from build123d import *

# Parameters (mm, degrees)
F0_R     = 4.1529
F1_DEPTH = 6.35
F2_R     = 5.08
F3_R     = 0.79375
F4_DEPTH = 6.604


with BuildPart() as f1:
    # F0 (on Top) → F1 (new body)
    with BuildSketch(Plane.XY):
        with BuildLine():
            Line((-39.5852921817, 35.7330972108), (-43.6584469102, 37.7552635994))
            ThreePointArc((-43.6584469102, 37.7552635994), (-77.757072432, 20.950769545), (-57.9630675112, -11.5038857774))
            Line((-57.9630675112, -11.5038857774), (-52.1653779445, -11.9667752425))
            ThreePointArc((-52.1653779445, -11.9667752425), (-34.5169287333, -4.1314539733), (-27.2771428081, 13.7695381418))
            ThreePointArc((-27.2771428081, 13.7695381418), (-30.5639418609, 26.3581090295), (-39.5852921817, 35.7330972108))
        make_face()
        with BuildLine():
            ThreePointArc((-39.5852921817, 35.7330972108), (-41.5771437171, 36.8342695403), (-43.6584469102, 37.7552635994))
            Line((-43.6584469102, 37.7552635994), (-39.5852921817, 35.7330972108))
        make_face()
        with BuildLine():
            Line((-52.1653779445, -11.9667752425), (-57.9630675112, -11.5038857774))
            ThreePointArc((-57.9630675112, -11.5038857774), (-55.0773333512, -11.8995410396), (-52.1653779445, -11.9667752425))
        make_face()
        with BuildLine():
            Line((0, 16.0805053817), (-39.5852921817, 35.7330972108))
            ThreePointArc((-39.5852921817, 35.7330972108), (-30.5639418609, 26.3581090295), (-27.2771428081, 13.7695381418))
            ThreePointArc((-27.2771428081, 13.7695381418), (-34.5169287333, -4.1314539733), (-52.1653779445, -11.9667752425))
            Line((-52.1653779445, -11.9667752425), (-1.2798007555, -16.0294966658))
            ThreePointArc((-1.2798007555, -16.0294966658), (-16.0677481424, 0.6404084366), (0, 16.0805053817))
        make_face()
        with BuildLine():
            ThreePointArc((12.550681619, 10.0530116996), (6.9615064675, 14.4955193434), (0, 16.0805053817))
            ThreePointArc((0, 16.0805053817), (-16.0677481424, 0.6404084366), (-1.2798007555, -16.0294966658))
            ThreePointArc((-1.2798007555, -16.0294966658), (10.9087765216, -11.8144508181), (16.0805053817, 0))
            ThreePointArc((16.0805053817, 0), (15.91872127, 2.2752948071), (15.4366243175, 4.5048066565))
            ThreePointArc((15.4366243175, 4.5048066565), (12.8528968999, 6.6855358941), (12.550681619, 10.0530116996))
        make_face()
        Circle(F0_R, mode=Mode.SUBTRACT)
        with BuildLine():
            ThreePointArc((21.2413206768, 8.7367389351), (17.4619629936, 13.1316161013), (12.550681619, 10.0530116996))
            ThreePointArc((12.550681619, 10.0530116996), (14.2659723887, 7.4205582766), (15.4366243175, 4.5048066565))
            ThreePointArc((15.4366243175, 4.5048066565), (19.4149247594, 5.1449514054), (21.2413206768, 8.7367389351))
        make_face()
        with BuildLine():
            ThreePointArc((15.4366243175, 4.5048066565), (14.2659723887, 7.4205582766), (12.550681619, 10.0530116996))
            ThreePointArc((12.550681619, 10.0530116996), (12.8528968999, 6.6855358941), (15.4366243175, 4.5048066565))
        make_face()
    extrude(amount=F1_DEPTH)

    # F2
    f2_edges = [f1.edges().sort_by_distance(p)[0] for p in [
        (12.550682, 10.053012, 3.175),
        (15.436624, 4.504807, 3.175),
        (0, 16.080505, 3.175),
    ]]
    fillet(f2_edges, radius=F2_R)

    # F3 (on face) → F4 (cut)
    with BuildSketch(Plane.XY.offset(6.35)):
        with Locations((16.7963206768, 8.7367389351)):
            Circle(F3_R)
    extrude(amount=-F4_DEPTH, mode=Mode.SUBTRACT)


solid = f1.part
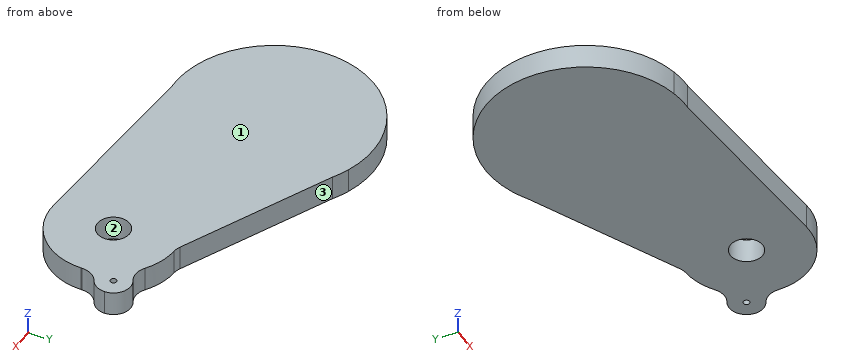
For this review, take the finished solid that the model builds, in its own axes (mm). Face numbers are marked on the shaded views. Give positions to 0.01 mm unless a question says otherwise; leave off trailing zeros. Order: outer loops, then holes, each group sorted by start corner. A loop starts at its lowest first (then second) coordinate and runs counter-clockwise, first axis right, second up. Notation, with made-up numbers: M 26.25,52.25 L 64.25,52.25 A25 ccw 64.25,86.25 Z; hole C 3,31.25 d9. An arc over 180 degrees is marked long. Answer in a Markdown table with one row per item. Add a question column.
(1) Consider section C-C on y = 28. State the section outline as (x, z) points.
(2) Consider section D-D on x = -50.5. State the section outline as (y, z) points.
(3) Wall thickness on probe 1 along X at (y, z) = (-3.5, 2.75); probe 2 along X at (y, z) = (12.5, 1.5); probe 3 along Y at (x, z) = (0, 1.5): over which ranges is each line inside the solid? List them lowest first. Write a range as [from, to].
(4) Mouldability with a two-part tool opening along X and no side actions: class the marked faces 1, 2 and 3 as +X half, -X half, draft (parallel to the pull), parting line (faces both ways), or undercut.
(5) Consider section A-A on x = 0. State the section outline as (y, z) points, and give its area (3 significant figures).
(6) For pin 1 (1.4 mm diameter, centred on x = 16.8, y = 8.74, fed in from +Z); pin 2 (3 mm diameter, centred on x = -15.5, z = 2, fed in from +Y); pin 3 (1 mm diameter, centred on x = -66.5, z = 4, fed in from -Y); pin 4 (1 mm diameter, centred on x = -65, z = 5, fed in from -Y), all flat-tipped, find the tip position at first contact; note any pin that passes through.
(7) Consider section B-B on z = 1. Give the number of separate pieces and of enclosed holes in the cut face, and give its area (3 significant figures).
Evaluation:
| question | item | result |
|---|---|---|
| 1 | outline | M -74.49,0 L -24.01,0 L -24.01,6.35 L -74.49,6.35 Z |
| 2 | outline | M -12.1,0 L 39.4,0 L 39.4,6.35 L -12.1,6.35 Z |
| 3 | probe 1 | x = [-72.13, -2.24], [2.24, 15.69] |
| 3 | probe 2 | x = [-78.75, 10.37], [14.37, 19.16] |
| 3 | probe 3 | y = [-16.08, -4.15], [4.15, 16.2] |
| 4 | face 1 | draft |
| 4 | face 2 | undercut |
| 4 | face 3 | +X half |
| 5 | outline | M -16.08,0 L -4.15,0 L -4.15,6.35 L -16.08,6.35 Z; M 4.15,0 L 16.2,0 L 16.2,6.35 L 4.15,6.35 Z |
| 5 | area | 152 mm^2 |
| 6 | pin 1 | passes through |
| 6 | pin 2 | stops at y = 24.52 |
| 6 | pin 3 | stops at y = -8.48 |
| 6 | pin 4 | stops at y = -9.28 |
| 7 | separate pieces | 1 |
| 7 | enclosed holes | 2 |
| 7 | area | 3,740 mm^2 |
